Autodesk Inventor part; units mm, degrees
ref_plane "Work Plane3" through (0, 3, 0) normal (0, -1, 0) x (1, 0, 0)
ref_plane "Work Plane4" through (0, 9, 0) normal (0, -1, 0) x (1, 0, 0)
ref_plane "Work Plane12" through (0, 15, 0) normal (0, -1, 0) x (1, 0, 0)
sketch "Sketch1" plane through (0, 0, 0) normal (0, 1, 0) x (-1, 0, 0)
  line L0 (22.5, 25) -> (-22.5, 25)
  line L1 (-22.5, 25) -> (-22.5, -25)
  line L2 (-22.5, -25) -> (22.5, -25)
  line L3 (22.5, -25) -> (22.5, 25)
  line L4 (22.5, 25) -> (-22.5, -25) construction
  line L5 (-22.5, 25) -> (22.5, -25) construction
  point P0 (0, 0)
  dimension "d0" = 45
  dimension "d1" = 50
extrude "Extrusion1" add sketch "Sketch1" along normal blind 60
fillet "Fillet1" radius 4 4 edges at (22.5, 30, 25) (-22.5, 30, 25) (22.5, 30, -25) (-22.5, 30, -25)
sketch "Sketch2" plane through (0, 60, 0) normal (0, 1, 0) x (1, 0, 0)
  circle A0 centre (0, 3) radius 16
  point P0 (0, 0)
  dimension "d5" = 32
  dimension "d109" = 3
extrude "Extrusion2" cut sketch "Sketch2" against normal blind 60
ref_plane "Work Plane3" through (0, 3, 0) normal (0, -1, 0) x (1, 0, 0)
sketch "Sketch13" plane through (0, 3, 0) normal (0, -1, 0) x (1, 0, 0)
  circle A0 centre (42, -3) radius 24
  point P0 (0, 0)
  dimension "d27" = 48
extrude "Extrusion7" cut sketch "Sketch13" against normal blind 3
ref_plane "Work Plane4" through (0, 9, 0) normal (0, -1, 0) x (1, 0, 0)
sketch "Sketch14" plane through (0, 9, 0) normal (0, -1, 0) x (1, 0, 0)
  circle A0 centre (42, -3) radius 24
  point P0 (0, 0)
  dimension "d34" = 48
extrude "Extrusion8" cut sketch "Sketch14" against normal blind 3
ref_plane "Work Plane12" through (0, 15, 0) normal (0, -1, 0) x (1, 0, 0)
sketch "Sketch15" plane through (0, 15, 0) normal (0, -1, 0) x (1, 0, 0)
  circle A0 centre (42, -3) radius 24
  point P0 (0, 0)
  dimension "d41" = 48
extrude "Extrusion9" cut sketch "Sketch15" against normal blind 3
ref_plane "Work Plane13" through (0, 21, 0) normal (0, -1, 0) x (1, 0, 0)
sketch "Sketch16" plane through (0, 21, 0) normal (0, -1, 0) x (1, 0, 0)
  arc A0 (22.5, 10.9911) -> (22.5, -16.9911) centre (42, -3) ccw
  circle A1 centre (42, -3) radius 24
  point P0 (0, 0)
  point P1 (22.5, -16.9911)
  dimension "d45" = 48
extrude "Extrusion10" cut sketch "Sketch16" against normal blind 3
ref_plane "Work Plane14" through (0, 27, 0) normal (0, -1, 0) x (1, 0, 0)
sketch "Sketch17" plane through (0, 27, 0) normal (0, -1, 0) x (1, 0, 0)
  circle A0 centre (42, -3) radius 24
  point P0 (0, 0)
  dimension "d49" = 48
extrude "Extrusion11" cut sketch "Sketch17" against normal blind 3
ref_plane "Work Plane15" through (0, 33, 0) normal (0, -1, 0) x (1, 0, 0)
sketch "Sketch18" plane through (0, 33, 0) normal (0, -1, 0) x (1, 0, 0)
  circle A0 centre (42, -3) radius 24
  point P0 (0, 0)
  dimension "d53" = 48
extrude "Extrusion12" cut sketch "Sketch18" against normal blind 3
ref_plane "Work Plane16" through (0, 39, 0) normal (0, -1, 0) x (1, 0, 0)
sketch "Sketch19" plane through (0, 39, 0) normal (0, -1, 0) x (1, 0, 0)
  circle A0 centre (42, -3) radius 24
  point P0 (0, 0)
  dimension "d57" = 48
extrude "Extrusion13" cut sketch "Sketch19" against normal blind 3
ref_plane "Work Plane17" through (0, 45, 0) normal (0, -1, 0) x (1, 0, 0)
sketch "Sketch20" plane through (0, 45, 0) normal (0, -1, 0) x (1, 0, 0)
  circle A0 centre (42, -3) radius 24
  point P0 (0, 0)
  dimension "d61" = 48
extrude "Extrusion14" cut sketch "Sketch20" against normal blind 3
ref_plane "Work Plane18" through (0, 51, 0) normal (0, -1, 0) x (1, 0, 0)
sketch "Sketch21" plane through (0, 51, 0) normal (0, -1, 0) x (1, 0, 0)
  circle A0 centre (42, -3) radius 24
  point P0 (0, 0)
  dimension "d65" = 48
extrude "Extrusion15" cut sketch "Sketch21" against normal blind 3
mirror "Mirror1" about plane through (0, 0, 0) normal (1, 0, 0) of "Extrusion7", "Extrusion8", "Extrusion9", "Extrusion10", "Extrusion11", "Extrusion12", "Extrusion13", "Extrusion14", "Extrusion15"
pattern_circular "Circular Pattern3" count 2 over 90 about axis through (0, 60, -3) along (0, 1, 0) of "Extrusion15", "Extrusion14", "Extrusion13", "Extrusion12", "Extrusion11", "Extrusion10", "Extrusion9", "Extrusion8", "Extrusion7"
sketch "Sketch22" plane through (0, 0, 0) normal (0, -1, 0) x (1, 0, 0)
  line L0 (2, 11) -> (-2, 11)
  line L1 (-2, 11) -> (-2, 21)
  line L2 (-2, 21) -> (2, 21)
  line L3 (2, 21) -> (2, 11)
  line L4 (2, 11) -> (-2, 21) construction
  line L5 (-2, 11) -> (2, 21) construction
  point P0 (0, 0)
  point P1 (0, 16)
  dimension "d74" = 4
  dimension "d75" = 10
extrude "Extrusion16" cut sketch "Sketch22" against normal blind 2
sketch "Sketch23" plane through (0, 0, 0) normal (0, -1, 0) x (1, 0, 0)
  line L0 (0, 0) -> (0, 21)
  line L1 (-2, 12.8745) -> (-2, 21)
sketch "Sketch24" plane through (0, 0, 0) normal (0, -1, 0) x (1, 0, 0)
  circle A0 centre (0, 21) radius 2
  point P0 (0, 0)
  dimension "d78" = 4
extrude "Extrusion17" cut sketch "Sketch24" against normal blind 62
sketch "Sketch25" plane through (0, 0, 21) normal (0, -1, 0) x (1, 0, 0)
  point P0 (0, -21)
sketch "Sketch27" plane through (0, 60, 0) normal (0, 1, 0) x (1, 0, 0)
  line L0 (0, 3) -> (-16.2635, 19.2635)
  line L1 (0, 3) -> (23, 3) construction
  circle A0 centre (-16.2635, 19.2635) radius 3.5
  point P0 (0, 0)
  dimension "d91" = 23
  dimension "d92" = 135
  dimension "d93" = 7
extrude "Extrusion18" cut sketch "Sketch27" against normal blind 60
pattern_circular "Circular Pattern5" count 4 over 360 about axis through (0, 60, -3) along (0, -1, 0) of "Extrusion18"
sketch "Sketch30" plane through (0, 60, 0) normal (0, 1, 0) x (1, 0, 0)
  circle A0 centre (0, 3) radius 18
  point P0 (0, 0)
  dimension "d110" = 36
extrude "Extrusion21" add sketch "Sketch30" along normal blind 2
sketch "Sketch31" plane through (0, 62, -3) normal (0, 1, 0) x (1, 0, 0)
  circle A0 centre (0, 0) radius 16
  point P0 (0, -3)
  dimension "d113" = 32
extrude "Extrusion22" cut sketch "Sketch31" against normal blind 2
properties part number "cylinder incomplete"
For this review, take the finished solid that the model builds, in its own axes (mm). A direction names the side the tool comes from. Coordinates: 2 decimals unless noted, no trailing zeros. Loops run counter-clockwise (first coordinate to the right, second up) from the corner with the lowest first, then second, coordinate; pieces in that order, holes last. Notation, with made-up numbers: (73.5, -10.5) - (91.5, -10.5) arc R31 cw to (91.5, 16.5) - close; hole circle Ø6 at (21, 43). An arc over 180 degrees is marked (long way). Use a Markdown table: item, result. Add a question column.
Item 1: We need section B-B (y = 46.5). Give the boundary of the cut face in (x, z).
Item 2: Tool access review of faces 1 (the face through (-21, 54, -3)), 2 (the face through (0, 2, 16)), 3 (the face through (21, 3, -3)), 4 (the face through (0, 27, -23)): name each direction out of +Z, -Z, +X, -X, +Y, -Y from which nothing blocks a thin tool from reaching the whole face with its end or side.
Item 3: We need section C-C (y = 58). Give the boundary of the cut face in (x, z).
Item 4: Insertion check: pin 1 Ø2.5 at (x, z) = (-21, 0.5) entering from +Y. The pin has a flat end and moves straight along its axis. Give the tip position at first contact, or say it passes through.
Item 5: Mouldability with a two-part tool opening along X and no side actions: class faces 5 (the face through (0, 40, -21)), 6 (the face through (18, 46, -3)), 7 (the face through (-21, 27, -3)) as pulls with the +X half, pulls with the -X half, needs draft (parallel to the pull), parting line crosses it, or undercut.
Item 6: We need section A-A (x = 0). Give the number of separate pieces and of enclosed holes in the cut face, and give its area (3 significant figures).
Item 7: For line 1 (Z direction, x = 16.5, y = 27.5); line 2 (X direction, y = 50, z = -3); line 3 (X direction, y = 24, z = 11), list the stretches that pass through material, from the lowest coordinate up.
Results list:
| question | item | result |
|---|---|---|
| 1 | outline | (-22.5, -21) arc R4 ccw to (-18.5, -25) - (-13.27, -25) arc R24 cw to (13.27, -25) - (18.5, -25) arc R4 ccw to (22.5, -21) - (22.5, -16.99) arc R24 cw to (22.5, 10.99) - (22.5, 21) arc R4 ccw to (18.5, 25) - (-18.5, 25) arc R4 ccw to (-22.5, 21) - (-22.5, 10.99) arc R24 cw to (-22.5, -16.99) - close; hole circle Ø7 at (-16.26, -19.26); hole circle Ø7 at (-16.26, 13.26); hole circle Ø32 at (0, -3); hole circle Ø4 at (0, 21); hole circle Ø7 at (16.26, -19.26); hole circle Ø7 at (16.26, 13.26) |
| 2 | face 1 | -X |
| 2 | face 2 | -Y |
| 2 | face 3 | +X |
| 2 | face 4 | -Z |
| 3 | outline | (-22.5, -21) arc R4 ccw to (-18.5, -25) - (18.5, -25) arc R4 ccw to (22.5, -21) - (22.5, 21) arc R4 ccw to (18.5, 25) - (-18.5, 25) arc R4 ccw to (-22.5, 21) - close; hole circle Ø7 at (-16.26, -19.26); hole circle Ø7 at (-16.26, 13.26); hole circle Ø32 at (0, -3); hole circle Ø4 at (0, 21); hole circle Ø7 at (16.26, -19.26); hole circle Ø7 at (16.26, 13.26) |
| 4 | pin 1 | stops at y = 60 |
| 5 | face 5 | undercut |
| 5 | face 6 | pulls with the +X half |
| 5 | face 7 | needs draft |
| 6 | separate pieces | 3 |
| 6 | enclosed holes | 0 |
| 6 | area | 728 mm^2 |
| 7 | line 1 | z = -25 to -22.76, -15.77 to 9.77, 16.76 to 25 |
| 7 | line 2 | x = -22.5 to -16, 16 to 22.5 |
| 7 | line 3 | x = -22.5 to -18.93, -13.59 to -7.75, 7.75 to 13.59, 18.93 to 22.5 |
